The model under review builds one solid part; all positions refer to its coordinate system, in mm. A direction names the side the tool comes from. Coordinates: 2 decimals unless noted, no trailing zeros. Write each loop counter-clockwise with the first axis right and the second up, starting at its lowest first coordinate (ties: lowest second). Pieces come first, ordered by that corner, then holes. Notation, with made-up numbers: (-25.75, 83.25) - (-8.75, 83.25) arc R28 ccw to (-8.75, 103.25) - close; hole circle Ø8 at (3, -28.75). An arc over 180 degrees is marked (long way). Return JSON: item names as keys, results as strings. Group by question number.
(1) We need section B-B on z = -0.5. State the section outline as (x, y) points.
(2) We need section A-A on y = 16.5. State the section outline as (x, z) points.
(3) For pin 1 Ø6.5 at (x, z) = (4.5, 12) entering from +Y, flat-tipped, find the tip position at first contact; note if it passes through.
(4) To check wall thickness, follow L1, parallel to Z at x = -13, y = 27.5; L2, parallel to Z at x = 0, y = 14.75; L3, parallel to Y at x = -2, z = 16.5. State the ranges of each line that lie inside material, in increasing order. Write a range as from..to.
(5) Draft analysis for pull direction X (two halves, no side actions). For faces 1 (the face through (0, 15, -6.512)), 2 (the face through (11.35, 17.32, 8.95)), 3 (the face through (-14.641, 15, 12)), state which applies: released by +X, released by -X, zero draft, split by the parting line, or undercut.
(6) Tool access review of faces 4 (the face through (1, 5, 9)), 5 (the face through (-13, 17, 9.988)), 6 (the face through (0, 15, 23.488)): name each direction out of +Z, -Z, +X, -X, +Y, -Y from which nothing blocks a thin tool from reaching the whole face with its end or side.
```python
from build123d import *

# Parameters (mm, degrees)
SKETCH1_W           = 30
SKETCH1_H           = 30
SKETCH1_R           = 11
BOSS_EXTRUDE1_DEPTH = 30
SKETCH2_W           = 1.5
SKETCH2_H           = 30
CUT_EXTRUDE1_DEPTH  = 11
SKETCH4_W           = 30
SKETCH4_H           = 30
BOSS_EXTRUDE3_DEPTH = 5


with BuildPart() as part:
    # Sketch1 → Boss-Extrude1 (new body)
    with BuildSketch(Plane(origin=(0, 0, 0), x_dir=(1, 0, 0), z_dir=(0, 1, 0))):
        with Locations((0.359281437, -8.488023952)):
            Rectangle(SKETCH1_W, SKETCH1_H)
        with Locations(Location((0.359281437, -8.488023952, 0), (0, 0, 270))):
            Circle(SKETCH1_R, mode=Mode.SUBTRACT)
    extrude(amount=BOSS_EXTRUDE1_DEPTH)

    # Sketch2 → Cut-Extrude1 (cut)
    with BuildSketch(Plane.ZY.offset(14.640718563)):
        with Locations((7.738023952, 15)):
            Rectangle(SKETCH2_W, SKETCH2_H)
        with Locations((9.238023952, 15)):
            Rectangle(SKETCH2_W, SKETCH2_H)
    extrude(amount=-CUT_EXTRUDE1_DEPTH, mode=Mode.SUBTRACT)

    # Sketch4 → Boss-Extrude3 (add)
    with BuildSketch(Plane.XZ):
        with Locations((0.359281437, 8.488023952)):
            Rectangle(SKETCH4_W, SKETCH4_H)
    extrude(amount=-BOSS_EXTRUDE3_DEPTH)


solid = part.part
```
Ans:
{
 "1": {"outline": "(-14.64, 0) - (15.36, 0) - (15.36, 30) - (6.7, 30) - (6.7, 5) - (-5.98, 5) - (-5.98, 30) - (-14.64, 30) - close"},
 "2": {"outline": "(-14.64, -6.51) - (15.36, -6.51) - (15.36, 23.49) - (-14.64, 23.49) - (-14.64, 9.99) - (-10.54, 9.99) arc R11 cw (long way) to (-10.54, 6.99) - (-14.64, 6.99) - close"},
 "3": {"pin 1": "y = 5"},
 "4": {"L1": "-6.51..6.99, 9.99..23.49", "L2": "-6.51..-2.51, 19.48..23.49", "L3": "0..5"},
 "5": {"face 1": "zero draft", "face 2": "undercut", "face 3": "released by -X"},
 "6": {"face 4": "+Y", "face 5": "-X, +Y", "face 6": "+Z, +X, -X, +Y, -Y"}
}
